Verification items for the finished model (mm, model axes). Face numbers are marked on the shaded views. A direction names the side the tool comes from. Give positions to 0.01 mm unless a question says otherwise; leave off trailing zeros. Loops run counter-clockwise (first coordinate to the right, second up) from the corner with the lowest first, then second, coordinate; pieces in that order, holes last. Notation, with made-up numbers: M 84.5,8 L 94.5,8 A12 ccw 94.5,28 Z; hole C 13,84.5 d3. An arc over 180 degrees is marked long. Put each result on its own line as item: value. Start each with the question number.
Autodesk Fusion 360 part; units mm, degrees
sketch "Sketch1" plane through (0, 0, 0) normal (0, 0, 1) x (1, 0, 0)
  line L0 (-6.3509, 11) -> (-12.7017, 0)
  line L1 (-12.7017, 0) -> (-6.3509, -11)
  line L2 (-6.3509, -11) -> (6.3509, -11)
  line L3 (6.3509, -11) -> (12.7017, 0)
  line L4 (12.7017, 0) -> (6.3509, 11)
  line L5 (6.3509, 11) -> (-6.3509, 11)
  dimension "d1" = 11
extrude "Extrude1" add sketch "Sketch1" along normal blind 6
fillet "Fillet1" radius 3 6 edges at (6.3509, -11, 3) (12.7017, 0, 3) (-6.3509, -11, 3) (-12.7017, 0, 3) (-6.3509, 11, 3) (6.3509, 11, 3)
sketch "Sketch2" plane through (0, 0, 0) normal (0, 0, -1) x (1, 0, 0)
  arc A0 (4.6188, -11) -> (7.2169, -9.5) centre (4.6188, -8) ccw
  line L0 (7.2169, -9.5) -> (11.8357, -1.5)
  arc A1 (11.8357, -1.5) -> (11.8357, 1.5) centre (9.2376, 0) ccw
  line L1 (11.8357, 1.5) -> (7.2169, 9.5) construction
  arc A2 (7.2169, 9.5) -> (4.6188, 11) centre (4.6188, 8) ccw
  line L2 (4.6188, 11) -> (-4.6188, 11)
  arc A3 (-4.6188, 11) -> (-7.2169, 9.5) centre (-4.6188, 8) ccw
  line L3 (-7.2169, 9.5) -> (-11.8357, 1.5)
  arc A4 (-11.8357, 1.5) -> (-11.8357, -1.5) centre (-9.2376, 0) ccw
  line L4 (-11.8357, -1.5) -> (-7.2169, -9.5)
  arc A5 (-7.2169, -9.5) -> (-4.6188, -11) centre (-4.6188, -8) ccw
  line L5 (-4.6188, -11) -> (4.6188, -11)
  line L6 (-8.0829, 10) -> (-12.7017, 2)
  arc A6 (-12.7017, 2) -> (-12.7017, -2) centre (-9.2376, 0) ccw
  line L7 (-12.7017, -2) -> (-8.0829, -10)
  arc A7 (-8.0829, -10) -> (-4.6188, -12) centre (-4.6188, -8) ccw
  line L8 (-4.6188, -12) -> (4.6188, -12)
  arc A8 (4.6188, -12) -> (8.0829, -10) centre (4.6188, -8) ccw
  line L9 (8.0829, -10) -> (12.7017, -2)
  arc A9 (12.7017, -2) -> (12.7017, 2) centre (9.2376, 0) ccw
  line L10 (12.7017, 2) -> (8.0829, 10)
  arc A10 (8.0829, 10) -> (4.6188, 12) centre (4.6188, 8) ccw
  line L11 (4.6188, 12) -> (-4.6188, 12)
  arc A11 (-4.6188, 12) -> (-8.0829, 10) centre (-4.6188, 8) ccw
  dimension "d6" = 1
extrude "Extrude2" add sketch "Sketch2" along normal blind 2
sketch "Sketch3" plane through (0, 0, 6) normal (0, 0, 1) x (-1, 0, 0)
  arc A0 (-7.2169, -9.5) -> (-4.6188, -11) centre (-4.6188, -8) ccw
  line L0 (-4.6188, -11) -> (4.6188, -11)
  arc A1 (4.6188, -11) -> (7.2169, -9.5) centre (4.6188, -8) ccw
  line L1 (7.2169, -9.5) -> (11.8357, -1.5) construction
  arc A2 (11.8357, -1.5) -> (11.8357, 1.5) centre (9.2376, 0) ccw
  line L2 (11.8357, 1.5) -> (7.2169, 9.5)
  arc A3 (7.2169, 9.5) -> (4.6188, 11) centre (4.6188, 8) ccw
  line L3 (4.6188, 11) -> (-4.6188, 11)
  arc A4 (-4.6188, 11) -> (-7.2169, 9.5) centre (-4.6188, 8) ccw
  line L4 (-7.2169, 9.5) -> (-11.8357, 1.5)
  arc A5 (-11.8357, 1.5) -> (-11.8357, -1.5) centre (-9.2376, 0) ccw
  line L5 (-11.8357, -1.5) -> (-7.2169, -9.5)
  line L6 (8.425, -0.6467) -> (5.7257, 0.0765)
  line L7 (5.6158, -2.5276) -> (4.0271, -2.1019)
  line L8 (5.7257, 0.0765) -> (2.4486, 5.7527)
  line L9 (-4.0271, 2.1019) -> (-8.3151, 3.2509)
  line L10 (-0.4766, -8.3268) -> (9.5251, -2.5523)
  line L11 (-9.5251, 2.5523) -> (-3.7506, -7.4495)
  line L12 (8.425, -0.6467) -> (3.7506, 7.4495)
  line L13 (-0.7558, -6.2062) -> (5.6158, -2.5276)
  line L14 (-4.9203, 2.9291) -> (-7.6196, 3.6524)
  line L15 (-8.3151, 3.2509) -> (-9.5251, 2.5523)
  line L16 (0.7558, 6.2062) -> (-4.9203, 2.9291)
  line L17 (0.4766, 8.3268) -> (-7.6196, 3.6524)
  line L18 (9.5251, -2.5523) -> (8.8265, -1.3422)
  line L19 (-6.1272, 0.6189) -> (-2.4486, -5.7527)
  line L20 (8.8265, -1.3422) -> (4.5385, -0.1932)
  line L21 (3.7506, 7.4495) -> (0.4766, 8.3268)
  line L22 (2.4486, 5.7527) -> (0.7558, 6.2062)
  line L23 (-0.7558, -6.2062) -> (-2.4486, -5.7527)
  line L24 (-0.4766, -8.3268) -> (-3.7506, -7.4495)
  circle A6 centre (0, 0) radius 1.9987
  circle A7 centre (0, 0) radius 3.9748
  arc A8 (-4.0271, 2.1019) -> (-4.5385, 0.1932) centre (0, 0) ccw
  line L25 (-4.5385, 0.1932) -> (-6.1272, 0.6189)
  arc A9 (4.0271, -2.1019) -> (4.5385, -0.1932) centre (0, 0) ccw
extrude "Extrude3" add sketch "Sketch3" along normal blind 1
chamfer "Chamfer1" distance 0.4 angle 45 36 edges at (9.5263, -5.5, 6) (12.2376, 0, 6) (9.5263, 5.5, 6) (6.1188, 10.5981, 6) (0, 11, 6) (-6.1188, 10.5981, 6) (-9.5263, 5.5, 6) (-12.2376, 0, 6) (-9.5263, -5.5, 6) (-6.1188, -10.5981, 6) (0, -11, 6) (6.1188, -10.5981, 6) (10.3923, -6, 0) (6.6188, -11.4641, 0) (0, -12, 0) (-6.6188, -11.4641, 0) (-10.3923, -6, 0) (-13.2376, 0, 0) (-10.3923, 6, 0) (-6.6188, 11.4641, 0) (0, 12, 0) (6.6188, 11.4641, 0) (10.3923, 6, 0) (13.2376, 0, 0) (10.3923, -6, -2) (6.6188, -11.4641, -2) (0, -12, -2) (-6.6188, -11.4641, -2) (-10.3923, -6, -2) (-13.2376, 0, -2) (-10.3923, 6, -2) (-6.6188, 11.4641, -2) (0, 12, -2) (6.6188, 11.4641, -2) (10.3923, 6, -2) (13.2376, 0, -2)
sketch "Sketch4" plane through (0, 0, -2) normal (0, 0, -1) x (1, 0, 0)
  line L0 (12.3553, 1.8) -> (7.7365, 9.8)
  arc A0 (7.7365, 9.8) -> (4.6188, 11.6) centre (4.6188, 8) ccw
  line L1 (4.6188, 11.6) -> (-4.6188, 11.6)
  arc A1 (-4.6188, 11.6) -> (-7.7365, 9.8) centre (-4.6188, 8) ccw
  line L2 (-7.7365, 9.8) -> (-12.3553, 1.8)
  arc A2 (-12.3553, 1.8) -> (-12.3553, -1.8) centre (-9.2376, 0) ccw
  line L3 (-12.3553, -1.8) -> (-7.7365, -9.8)
  arc A3 (-7.7365, -9.8) -> (-4.6188, -11.6) centre (-4.6188, -8) ccw
  line L4 (-4.6188, -11.6) -> (4.6188, -11.6)
  arc A4 (4.6188, -11.6) -> (7.7365, -9.8) centre (4.6188, -8) ccw
  line L5 (7.7365, -9.8) -> (12.3553, -1.8)
  arc A5 (12.3553, -1.8) -> (12.3553, 1.8) centre (9.2376, 0) ccw
  line L6 (0, 0) -> (-6.4188, -11.1177) construction
  line L7 (-3.2094, -5.5588) -> (1.5717, -4.2778)
  line L8 (1.5717, -4.2778) -> (-0.1604, -3.2778)
  line L9 (-0.1604, -3.2778) -> (2.8396, 1.9184)
  line L10 (2.8396, 1.9184) -> (1.5406, 2.6684)
  line L11 (1.5406, 2.6684) -> (0, 0) construction
  line L12 (-3.2094, -5.5588) -> (-4.4905, -0.7778)
  line L13 (-4.4905, -0.7778) -> (-2.7584, -1.7778)
  line L14 (0.2416, 3.4184) -> (1.5406, 2.6684)
  line L15 (-2.7584, -1.7778) -> (0.2416, 3.4184)
  dimension "d14" = 1.5
  dimension "d15" = 2
  dimension "d16" = 45
  dimension "d17" = 6
extrude "Extrude4" cut sketch "Sketch4" against normal blind 0.4 contours L7 L8 L9 L10 L12 L13 L14 L15
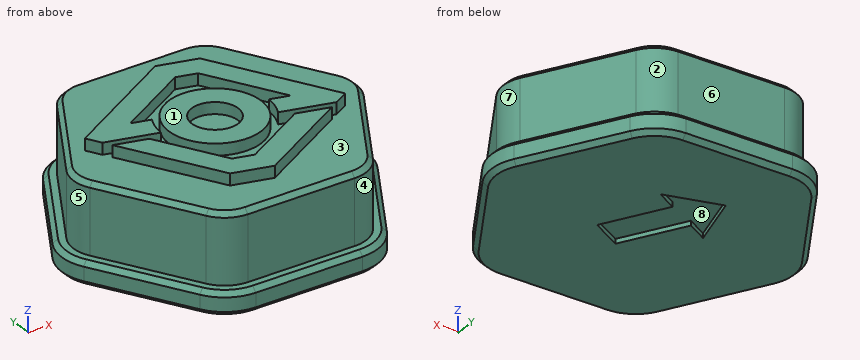
Q1. Release check for a two-part mould opening along X. For the marked faces 1, 2 and 3 record: pulls with the +X half, pulls with the -X half, needs draft (parallel to the pull), parting line crosses it, or undercut.
Q2. Cross-section at B-B, the plane x = 3.25. Record the boundary of the cut face in (y, z), then the cut area to 3 significant figures.
Q3. Cross-section at A-A, the plane z = 2.5. Record the boundary of the cut face in (x, y), then the cut area to 3 significant figures.
Q4. Set-up check for the marked faces 4, 5, 6, 7 and 8: record each of +Z, -Z, +X, -X, +Y, -Y from which the full face is reachable in a straight line by a thin tool's end or side.
Q5. Scan lines: L1, parallel to Y at x = 0, z = 6.55; L2, parallel to Z at x = -8.5, y = -1.25; L3, parallel to Z at x = 9.75, y = 6.25. Record each from-to range of solid material in increasing order.
Q6. Go/stop test with flat-tipped pins: pin 1 (4.5 mm diameter, centred on x = -1.5, z = 2, fed in from -Y); pin 2 (1 mm diameter, centred on y = 5, z = 1, fed in from -X); pin 3 (5 mm diameter, centred on x = 4, z = 4.5, fed in from -Y). Record where each tip stops, or that it passes through.
Ans:
1. face 1: needs draft
1. face 2: pulls with the +X half
1. face 3: undercut
2. outline: M -12,-1.6 L -11.6,-2 L 11.6,-2 L 12,-1.6 L 12,-0.4 L 11.6,0 L 11,0 L 11,5.6 L 10.6,6 L 7.58,6 L 7.58,7 L 4.36,7 L 4.36,6 L 2.29,6 L 2.29,7 L -2.29,7 L -2.29,6 L -3.89,6 L -3.89,7 L -6.18,7 L -6.18,6 L -10.6,6 L -11,5.6 L -11,0 L -11.6,0 L -12,-0.4 Z
2. area: 190 mm^2
3. outline: M -11.84,-1.5 L -7.22,-9.5 A3 ccw -4.62,-11 L 4.62,-11 A3 ccw 7.22,-9.5 L 11.84,-1.5 A3 ccw 11.84,1.5 L 7.22,9.5 A3 ccw 4.62,11 L -4.62,11 A3 ccw -7.22,9.5 L -11.84,1.5 A3 ccw Z
3. area: 416 mm^2
4. face 4: +Z, +X, -Y
4. face 5: +Z, -X
4. face 6: +Z, +X, -X, +Y
4. face 7: +Z, +X
4. face 8: -Z
5. L1: y = -8.05 to -5.77, -3.97 to -2, 2 to 3.97, 5.77 to 8.05
5. L2: z = -2 to 6
5. L3: z = -2 to 0
6. pin 1: stops at y = -11.85
6. pin 2: stops at x = -10.1
6. pin 3: stops at y = -11
